Source: CAD feature listing. Evaluate the final solid. Frame: model axes, mm. Face numbers are marked on the shaded views. A direction names the side the tool comes from. Give positions to 0.01 mm unless a question says otherwise; leave off trailing zeros. Order: outer loops, then holes, each group sorted by start corner. A loop starts at its lowest first (then second) coordinate and runs counter-clockwise, first axis right, second up. Notation, with made-up numbers: (-23.75, 75.5) - (-14.75, 75.5) arc R10 cw to (-14.75, 91.5) - close; hole circle Ø3 at (19.5, 41). An arc over 180 degrees is marked (long way). One line per item, written item: value. Start each with the question number.
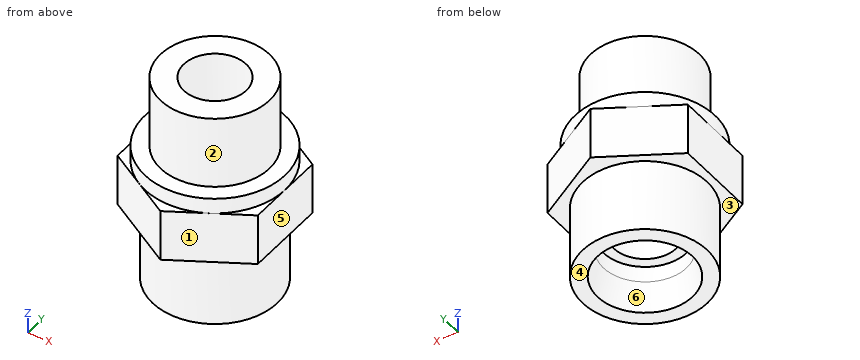
from build123d import *

# Parameters (mm, degrees)
BASE_EXTRUDE_DEPTH  = 10
SKETCH2_R           = 13.5
BOSS_EXTRUDE1_DEPTH = 3
SKETCH3_R           = 10.4775
BOSS_EXTRUDE2_DEPTH = 14
SKETCH4_R           = 12
BOSS_EXTRUDE3_DEPTH = 14
SKETCH5_R           = 6
CUT_EXTRUDE1_DEPTH  = 42


with BuildPart() as part:
    # Sketch1 → Base-Extrude (new body)
    with BuildSketch(Plane.XY):
        Polygon((0, 15.588457268), (-13.5, 7.794228634), (-13.5, -7.794228634), (0, -15.588457268), (13.5, -7.794228634), (13.5, 7.794228634), align=None)
    extrude(amount=BASE_EXTRUDE_DEPTH)

    # Sketch2 → Boss-Extrude1 (add)
    with BuildSketch(Plane.XY.offset(10)):
        Circle(SKETCH2_R)
    extrude(amount=BOSS_EXTRUDE1_DEPTH)

    # Sketch3 → Boss-Extrude2 (add)
    with BuildSketch(Plane.XY.offset(13)):
        Circle(SKETCH3_R)
    extrude(amount=BOSS_EXTRUDE2_DEPTH)

    # Sketch4 → Boss-Extrude3 (add)
    with BuildSketch(Plane(origin=(0, 0, 0), x_dir=(-1, 0, 0), z_dir=(0, 0, -1))):
        Circle(SKETCH4_R)
    extrude(amount=BOSS_EXTRUDE3_DEPTH)

    # Sketch5 → Cut-Extrude1 (cut, through all)
    with BuildSketch(Plane.XY.offset(27)):
        Circle(SKETCH5_R)
    extrude(amount=-CUT_EXTRUDE1_DEPTH, mode=Mode.SUBTRACT)

    # Sketch7 → Cut-Revolve1 (revolve, cut)
    with BuildSketch(Plane(origin=(0, 0, 0), x_dir=(0, 0, -1), z_dir=(1, 0, 0))):
        Polygon((14, 0), (14, 9.15), (8.589675374, 8), (5.5, 8), (5.5, 0), align=None)
    revolve(axis=Axis((0, 0, 0), (0, 0, -1)), mode=Mode.SUBTRACT)


solid = part.part
1. Contact query for flat-ended pins moving along their axis: pin 1 Ø1.5 at (x, z) = (-8.5, -9.5) entering from +Y; pin 2 Ø1.2 at (x, y) = (0.5, 13) entering from +Z; pin 3 Ø1 at (x, y) = (2.5, -3.5) entering from -Z; pin 4 Ø6 at (y, z) = (4.5, -3.5) entering from +X. Output: stop coordinate, or through.
2. Section D-D on z = 20.5. Return the cut outline in (x, y) (1 decimal), then the cut area to 3 significant figures.
3. Draft query along X for the marked faces 4, 5 and 6. Return one class per face: pulls with the +X half, pulls with the -X half, needs draft (parallel to the pull), parting line crosses it, or undercut.
4. Section C-C on y = 12.5. Return the cut outline in (x, z).
5. Section A-A on z = 5. Return the cut outline in (x, y), then the cut area to 3 significant figures.
6. Set-up query: the marked faces 1, 2 and 3. Return all of +Z, -Z, +X, -X, +Y, -Y with unobstructed straight access to the full face (end or side cutting, diameter ignored); none if empty.
7. Section B-B on x = -9.75. Return the cut outline in (y, z), then the cut area to 3 significant figures.
8. Ray query, L1, parallel to Y at x = 0, z = 5.5; L2, parallel to Z at x = -6.5, y = 0.5; L3, parallel to Z at x = -10.25, y = -9. Return the intervals inside material, ascending.
Data:
1. pin 1: stops at y = 9.16
1. pin 2: stops at z = 13
1. pin 3: passes through
1. pin 4: stops at x = 11.91
2. outline: circle Ø21 at (0, 0); hole circle Ø12 at (0, 0)
2. area: 232 mm2
3. face 4: needs draft
3. face 5: pulls with the +X half
3. face 6: undercut
4. outline: (-5.35, 0) - (5.35, 0) - (5.35, 10) - (5.1, 10) - (5.1, 13) - (-5.1, 13) - (-5.1, 10) - (-5.35, 10) - close
5. outline: (-13.5, -7.79) - (0, -15.59) - (13.5, -7.79) - (13.5, 7.79) - (0, 15.59) - (-13.5, 7.79) - close; hole circle Ø12 at (0, 0)
5. area: 518 mm2
6. face 1: +Z, -Z, +X, -Y
6. face 2: +Z
6. face 3: -Z
7. outline: (-9.96, 0) - (-7, 0) - (-7, -14) - (7, -14) - (7, 0) - (9.96, 0) - (9.96, 10) - (9.34, 10) - (9.34, 13) - (3.84, 13) - (3.84, 27) - (-3.84, 27) - (-3.84, 13) - (-9.34, 13) - (-9.34, 10) - (-9.96, 10) - close
7. area: 558 mm2
8. L1: y = -15.59 to -6, 6 to 15.59
8. L2: z = -5.5 to 27
8. L3: z = 0 to 10
